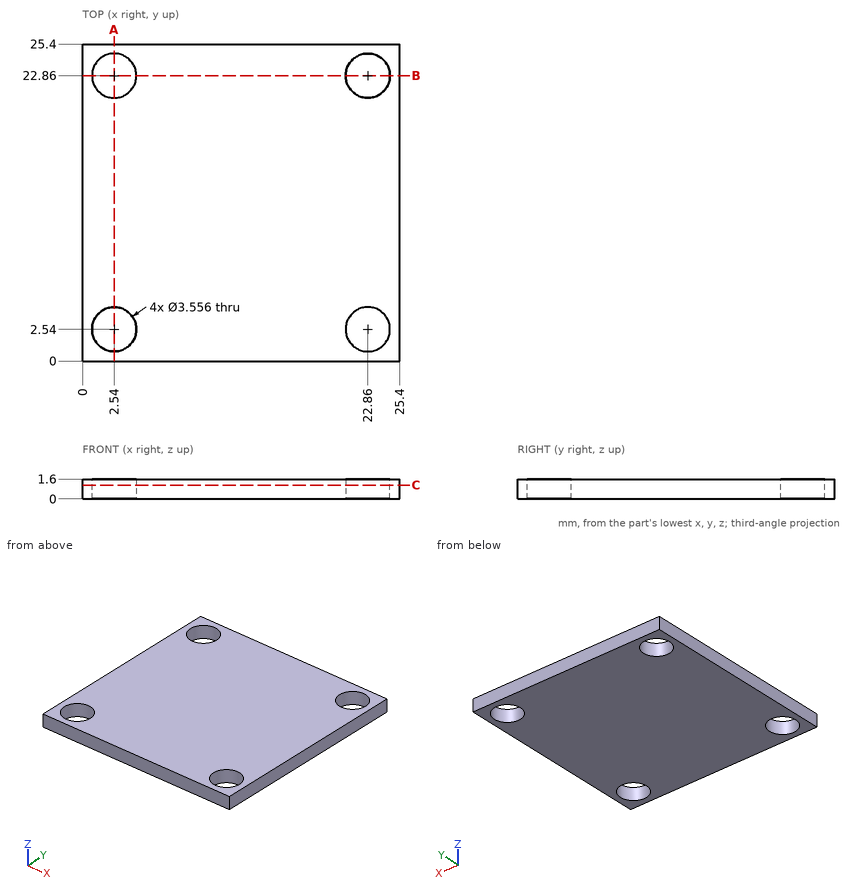
Source: three-view drawing plus pictorial views. Frame: mm from the lowest corner of the part. Round coordinates to 2 decimals unless told otherwise and drop trailing zeros. Order: outer loops, then holes, each group sorted by start corner. A loop starts at its lowest first (then second) coordinate and runs counter-clockwise, first axis right, second up. Notation, with made-up numbers: (87, 38) -> (98, 38) arc R14 cw to (98, 54) -> close; hole circle Ø9 at (32.25, -1.75). An arc over 180 degrees is marked (long way). Use one line per item in the form item = value.
(1) Section A-A on x = 2.54. Return loops of the section in (y, z), and give its area (3 significant figures).
Results list:
outline = (0, 0) -> (0.76, 0) -> (0.76, 1.6) -> (0, 1.6) -> close; (4.32, 0) -> (21.08, 0) -> (21.08, 1.6) -> (4.32, 1.6) -> close; (24.64, 0) -> (25.4, 0) -> (25.4, 1.6) -> (24.64, 1.6) -> close
area = 29.3 mm^2
(2) Section C-C on z = 1.1. Return loops of the section in (x, y), and give its area (3 significant figures).
Results list:
outline = (0, 0) -> (25.4, 0) -> (25.4, 25.4) -> (0, 25.4) -> close; hole circle Ø3.56 at (2.54, 2.54); hole circle Ø3.56 at (2.54, 22.86); hole circle Ø3.56 at (22.86, 2.54); hole circle Ø3.56 at (22.86, 22.86)
area = 605 mm^2
(3) Ray query, probe 1 along Y at (x, z) = (2.54, 0.4); probe 2 along X at (y, z) = (1, 0.4); probe 3 along Y at (x, z) = (1.25, 0.9). Return the intervals inside material, ascending. Write a range as [from, to].
Results list:
probe_1 = [0, 0.76], [4.32, 21.08], [24.64, 25.4]
probe_2 = [0, 1.65], [3.43, 21.97], [23.75, 25.4]
probe_3 = [0, 1.32], [3.76, 21.64], [24.08, 25.4]
